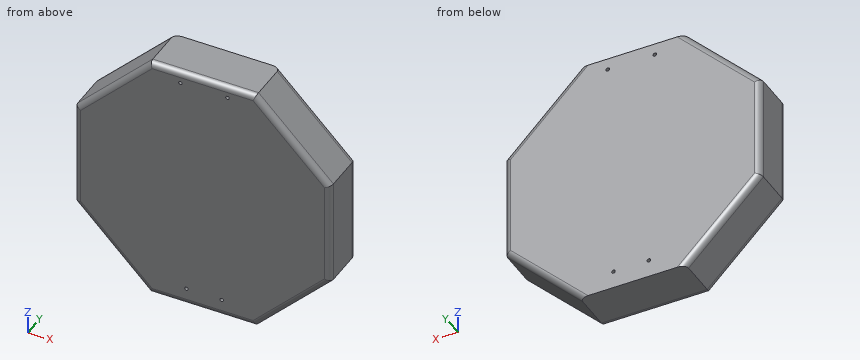
Autodesk Inventor part; units mm, degrees
ref_plane "YZ Plane" through (0, 0, 0) normal (1, 0, 0) x (0, 1, 0)
ref_plane "XZ Plane" through (0, 0, 0) normal (0, 1, 0) x (-1, 0, 0)
ref_plane "XY Plane" through (0, 0, 0) normal (0, 0, 1) x (1, 0, 0)
sketch "Эскиз1" plane through (0, 0, 0) normal (0, 1, 0) x (-1, 0, 0)
  line L0 (108.6396, 45) -> (108.6396, -45)
  line L1 (108.6396, -45) -> (45, -108.6396)
  line L2 (45, -108.6396) -> (-45, -108.6396)
  line L3 (-45, -108.6396) -> (-108.6396, -45)
  line L4 (-108.6396, -45) -> (-108.6396, 45)
  line L5 (-108.6396, 45) -> (-45, 108.6396)
  line L6 (-45, 108.6396) -> (45, 108.6396)
  line L7 (45, 108.6396) -> (108.6396, 45)
  point P0 (0, 0)
  point P1 (0, 0)
  dimension "d0" = 90
extrude "Выдавливание1" add sketch "Эскиз1" along normal blind 40
sketch "Эскиз2" plane through (0, 40, 0) normal (0, 1, 0) x (1, 0, 0)
  line L0 (-108.6396, 45) -> (-108.6396, -45)
  line L1 (-108.6396, -45) -> (-45, -108.6396)
  line L2 (-45, -108.6396) -> (45, -108.6396)
  line L3 (45, -108.6396) -> (108.6396, -45)
  line L4 (108.6396, -45) -> (108.6396, 45)
  line L5 (108.6396, 45) -> (45, 108.6396)
  line L6 (45, 108.6396) -> (-45, 108.6396)
  line L7 (-45, 108.6396) -> (-108.6396, 45)
  point P0 (0, 0)
  point P1 (-18.8883, -98.6396)
  point P2 (21.1117, -98.6396)
  point P3 (-13.7506, 93.6396)
  point P4 (16.2494, 93.6396)
  dimension "d3" = 40
  dimension "d4" = 10
  dimension "d12" = 30
  dimension "d13" = 15
hole "Отверстие1" at (-18.8883, 40, 98.6396) at (21.1117, 40, 98.6396) at (-13.7506, 40, -93.6396) at (16.2494, 40, -93.6396) direction (0, -1, 0) diameter 3 end through all
fillet "Сопряжение1" radius 5 14 edges at (-76.8198, 40, 76.8198) (-108.6396, 40, 0) (-76.8198, 40, -76.8198) (76.8198, 40, 76.8198) (108.6396, 40, 0) (76.8198, 40, -76.8198) (76.8198, 0, -76.8198) (108.6396, 0, 0) (76.8198, 0, 76.8198) (0, 0, -108.6396) (-76.8198, 0, -76.8198) (-108.6396, 0, 0) (-76.8198, 0, 76.8198) (0, 0, 108.6396)
properties part number "stand_bottom"
Could you check a few things on this model? Use its own coordinates, in mm. Round coordinates to 2 decimals unless told otherwise and drop trailing zeros. Write each loop counter-clockwise with the first axis right and the second up, starting at its lowest first coordinate (ties: lowest second). Pieces come first, ordered by that corner, then holes. Notation, with made-up numbers: M 65.5,10 L 111.5,10 A9 cw 111.5,20 Z; hole C -40,45 d6. An arc over 180 degrees is marked long. Answer in a Markdown table with one row per item. Add a question column.
Q1. Imagine slicing it at A-A (y = 9). Please give me the cut outline in (x, z).
Q2. If I drill on line 1 (Z direction, x = -19, y = 27.5); line 2 (Z direction, x = -85.5, y = 32); line 3 (Z direction, x = 72.5, y = 5), over which ranges is the centre line in solid material (lowest first)? Write a range as from..to.
Q3. Will these pins go through, and if not, where does the flat tip stop? pin 1 Ø1 at (y, z) = (29.5, 84) entering from -X; pin 2 Ø10 at (x, y) = (61.5, 27) entering from +Z; pin 3 Ø8 at (x, z) = (-37, -87) entering from -Y; pin 4 Ø6 at (x, y) = (-69.5, 7) entering from -Z.
Values:
| question | item | result |
|---|---|---|
| 1 | outline | M -108.64,-45 L -45,-108.64 L 45,-108.64 L 108.64,-45 L 108.64,45 L 45,108.64 L -45,108.64 L -108.64,45 Z; hole C -18.89,98.64 d3; hole C -13.75,-93.64 d3; hole C 16.25,-93.64 d3; hole C 21.11,98.64 d3 |
| 2 | line 1 | -108.64..97.14, 100.14..108.64 |
| 2 | line 2 | -68.14..68.14 |
| 2 | line 3 | -81.14..81.14 |
| 3 | pin 1 | x = -70.14 |
| 3 | pin 2 | z = 97.14 |
| 3 | pin 3 | y = 0 |
| 3 | pin 4 | z = -87.14 |
